```python
from build123d import *

# Parameters (mm, degrees)
SKETCH1_W            = 80.2
SKETCH1_H            = 80.2
BOSS_EXTRUDE1_DEPTH  = 4.5
M5_CLEARANCE_HOLE1_D = 5.5
SKETCH3_W            = 40
SKETCH3_H            = 4.5
BOSS_EXTRUDE2_DEPTH  = 30
CUT_EXTRUDE1_REACH   = 92.766
SKETCH4_R            = 5.25
CUT_EXTRUDE2_REACH   = 92.766
SKETCH5_R            = 1.924517265
FILLET2_R            = 10
FILLET4_R            = 5
FILLET3_R            = 5
CUT_EXTRUDE3_REACH   = 92.766
SKETCH6_R            = 11.25
FILLET5_R            = 5


with BuildPart() as part:
    # Sketch1 → Boss-Extrude1 (new body)
    with BuildSketch(Plane.XY):
        Rectangle(SKETCH1_W, SKETCH1_H)
    extrude(amount=BOSS_EXTRUDE1_DEPTH)

    # M5 Clearance Hole1 (through all)
    with Locations(Plane(origin=(-30.1, -30.1, 0), x_dir=(-1, 0, 0), z_dir=(0, 0, -1))):
        with Locations((0, 0), (-60.2, 60.2), (0, 60.2), (-60.2, 0)):
            Hole(M5_CLEARANCE_HOLE1_D / 2)

    # Sketch3 → Boss-Extrude2 (add)
    with BuildSketch(Plane(origin=(0, 0, 0), x_dir=(-1, 0, 0), z_dir=(0, 0, -1))):
        with Locations((0, 37.85)):
            Rectangle(SKETCH3_W, SKETCH3_H)
    extrude(amount=BOSS_EXTRUDE2_DEPTH)

    # Sketch4 → Cut-Extrude1 (cut, up to next)
    with BuildSketch(Plane(origin=(0, 35.6, 0), x_dir=(-1, 0, 0), z_dir=(0, -1, 0)), mode=Mode.PRIVATE) as cut_extrude1_sk1:
        with Locations(Location((0, 15, 0), (0, 0, 90))):
            Circle(SKETCH4_R)
    cut_extrude1_tool1 = extrude(cut_extrude1_sk1.sketch, amount=-CUT_EXTRUDE1_REACH, mode=Mode.PRIVATE) & part.part
    add(cut_extrude1_tool1.solids().sort_by_distance((0, 35.6, -15))[0], mode=Mode.SUBTRACT)

    # Sketch5 → Cut-Extrude2 (cut, up to next)
    with BuildSketch(Plane.XZ.offset(-35.6), mode=Mode.PRIVATE) as cut_extrude2_sk1:
        with Locations(Location((0, -23, 0), (0, 0, 270))):
            Circle(SKETCH5_R)
    cut_extrude2_tool1 = extrude(cut_extrude2_sk1.sketch, amount=-CUT_EXTRUDE2_REACH, mode=Mode.PRIVATE) & part.part
    # Sketch5 → Cut-Extrude2 (cut, up to next)
    with BuildSketch(Plane.XZ.offset(-35.6), mode=Mode.PRIVATE) as cut_extrude2_sk2:
        with Locations(Location((-8, -15, 0), (0, 0, 270))):
            Circle(SKETCH5_R)
    cut_extrude2_tool2 = extrude(cut_extrude2_sk2.sketch, amount=-CUT_EXTRUDE2_REACH, mode=Mode.PRIVATE) & part.part
    # Sketch5 → Cut-Extrude2 (cut, up to next)
    with BuildSketch(Plane.XZ.offset(-35.6), mode=Mode.PRIVATE) as cut_extrude2_sk3:
        with Locations(Location((0, -7, 0), (0, 0, 270))):
            Circle(SKETCH5_R)
    cut_extrude2_tool3 = extrude(cut_extrude2_sk3.sketch, amount=-CUT_EXTRUDE2_REACH, mode=Mode.PRIVATE) & part.part
    # Sketch5 → Cut-Extrude2 (cut, up to next)
    with BuildSketch(Plane.XZ.offset(-35.6), mode=Mode.PRIVATE) as cut_extrude2_sk4:
        with Locations(Location((8, -15, 0), (0, 0, 270))):
            Circle(SKETCH5_R)
    cut_extrude2_tool4 = extrude(cut_extrude2_sk4.sketch, amount=-CUT_EXTRUDE2_REACH, mode=Mode.PRIVATE) & part.part
    add(cut_extrude2_tool1.solids().sort_by_distance((0, 35.6, -23))[0], mode=Mode.SUBTRACT)
    add(cut_extrude2_tool2.solids().sort_by_distance((-8, 35.6, -15))[0], mode=Mode.SUBTRACT)
    add(cut_extrude2_tool3.solids().sort_by_distance((0, 35.6, -7))[0], mode=Mode.SUBTRACT)
    add(cut_extrude2_tool4.solids().sort_by_distance((8, 35.6, -15))[0], mode=Mode.SUBTRACT)

    # Fillet2
    fillet2_edges = [part.edges().sort_by_distance(p)[0] for p in [
        (40.1, -40.1, 2.25),
        (-40.1, -40.1, 2.25),
        (-40.1, 40.1, 2.25),
        (40.1, 40.1, 2.25),
    ]]
    fillet(fillet2_edges, radius=FILLET2_R)

    # Fillet4
    fillet4_edges = [part.edges().sort_by_distance(p)[0] for p in [
        (0, 35.6, 0),
    ]]
    fillet(fillet4_edges, radius=FILLET4_R)

    # Fillet3
    fillet3_edges = [part.edges().sort_by_distance(p)[0] for p in [
        (-20, 37.85, -30),
        (20, 37.85, -30),
    ]]
    fillet(fillet3_edges, radius=FILLET3_R)

    # Sketch6 → Cut-Extrude3 (cut, up to next)
    with BuildSketch(Plane.XZ.offset(-35.6), mode=Mode.PRIVATE) as cut_extrude3_sk1:
        with Locations((0, -15)):
            Circle(SKETCH6_R)
    cut_extrude3_tool1 = extrude(cut_extrude3_sk1.sketch, amount=CUT_EXTRUDE3_REACH, mode=Mode.PRIVATE) & part.part
    add(cut_extrude3_tool1.solids().sort_by_distance((0, 35.6, -15))[0], mode=Mode.SUBTRACT)

    # Fillet5
    fillet5_edges = [part.edges().sort_by_distance(p)[0] for p in [
        (-20, 35.35, 0),
        (20, 35.35, 0),
    ]]
    fillet(fillet5_edges, radius=FILLET5_R)


solid = part.part
```
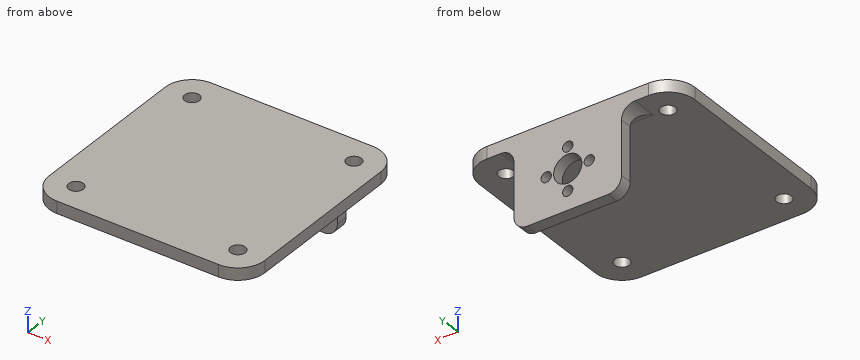
Part model, mm, in its own coordinate system. Round coordinates to 2 decimals unless told otherwise and drop trailing zeros. Write each loop counter-clockwise with the first axis right and the second up, starting at its lowest first coordinate (ties: lowest second). Pieces come first, ordered by that corner, then holes. Notation, with made-up numbers: M 1,47.5 L 43,47.5 A27 ccw 43,86.5 Z; hole C 23.5,89.25 d8. An arc over 180 degrees is marked long. One line per question, with ' | ' between items.
(1) Saw through at D-D on z = -11. Write the cut outline in (x, y).
Answer key:
outline: M -20,35.6 L -3.4,35.6 L -3.4,40.1 L -20,40.1 Z; M 3.4,35.6 L 20,35.6 L 20,40.1 L 3.4,40.1 Z
(2) Pin check, flat tips, straight feed: pin 1 (6 mm diameter, centred on x = -30, y = 20.5, fed in from -Z); pin 2 (1.5 mm diameter, centred on x = 20, z = -21, fed in from -Y); pin 3 (1.3 mm diameter, centred on y = 37, z = -18, fed in from -X). Stop position of each tip, or through.
Answer key:
pin 1: stops at z = 0 | pin 2: stops at y = 35.6 | pin 3: stops at x = -20
(3) Saw through at B-B on z = -23. Write the cut outline in (x, y).
Answer key:
outline: M -20,35.6 L -1.92,35.6 L -1.92,40.1 L -20,40.1 Z; M 1.92,35.6 L 20,35.6 L 20,40.1 L 1.92,40.1 Z
(4) Probe line 1 along Y through (x, z) = (-30.1, 3.2); line 2 along X through (y, z) = (37.3, -15); line 3 along X through (y, z) = (39.15, -7). List the from-to ranges inside material, lowest first.
Answer key:
line 1: y = -40.1 to -32.85, -27.35 to 27.35, 32.85 to 40.1 | line 2: x = -20 to -9.92, -6.08 to -5.25, 5.25 to 6.08, 9.92 to 20 | line 3: x = -20 to -1.92, 1.92 to 20
(5) Saw through at C-C on y = 20.5. Write the cut outline in (x, z).
Answer key:
outline: M -40.1,0 L 40.1,0 L 40.1,4.5 L -40.1,4.5 Z
(6) Saw through at A-A on x = 8. Write the cut outline in (y, z), then the cut area to 3 significant figures.
Answer key:
outline: M -40.1,0 L 30.6,0 A5 cw 35.6,-5 L 35.6,-13.08 L 40.1,-13.08 L 40.1,4.5 L -40.1,4.5 Z; M 35.6,-30 L 40.1,-30 L 40.1,-16.92 L 35.6,-16.92 Z | area: 484 mm^2
